```python
from build123d import *

# Parameters (mm, degrees)
SKETCH1_W           = 54
SKETCH1_H           = 44.4
SKETCH1_W_2         = 28
SKETCH1_H_2         = 6
BOSS_EXTRUDE1_DEPTH = 1.5
SKETCH2_R           = 1.5
SKETCH2_R_2         = 1
CUT_EXTRUDE1_DEPTH  = 1.5
BOSS_EXTRUDE2_DEPTH = 8
SKETCH4_R           = 7.5
BOSS_EXTRUDE3_DEPTH = 6
SKETCH5_R           = 5.877121991
BOSS_EXTRUDE4_DEPTH = 2
SKETCH6_R           = 7.5
BOSS_EXTRUDE5_DEPTH = 4
SKETCH7_R           = 5.097427656
CUT_EXTRUDE3_DEPTH  = 2
CHAMFER1_SIZE       = 2
BOSS_EXTRUDE6_DEPTH = 10
SKETCH9_W           = 9
SKETCH9_H           = 21
BOSS_EXTRUDE7_DEPTH = 10


with BuildPart() as part:
    # Sketch1 → Boss-Extrude1 (new body)
    with BuildSketch(Plane(origin=(0, 0, 0), x_dir=(1, 0, 0), z_dir=(0, 1, 0))):
        Rectangle(SKETCH1_W, SKETCH1_H)
        with Locations((0, -25.2)):
            Rectangle(SKETCH1_W_2, SKETCH1_H_2)
    extrude(amount=BOSS_EXTRUDE1_DEPTH)

    # Sketch2 → Cut-Extrude1 (cut)
    with BuildSketch(Plane(origin=(0, 1.5, 0), x_dir=(1, 0, 0), z_dir=(0, 1, 0))):
        with Locations(Location((-24, 19.2, 0), (0, 0, 270))):
            Circle(SKETCH2_R)
        with Locations(Location((24, 19.2, 0), (0, 0, 270))):
            Circle(SKETCH2_R)
        with Locations(Location((-24, -14.2, 0), (0, 0, 270))):
            Circle(SKETCH2_R)
        with Locations(Location((-10, -25.2, 0), (0, 0, 270))):
            Circle(SKETCH2_R)
        with Locations(Location((10, -25.2, 0), (0, 0, 270))):
            Circle(SKETCH2_R)
        with Locations(Location((0, 11.7, 0), (0, 0, 270))):
            Circle(SKETCH2_R_2)
    extrude(amount=-CUT_EXTRUDE1_DEPTH, mode=Mode.SUBTRACT)

    # Sketch3 → Boss-Extrude2 (add)
    with BuildSketch(Plane(origin=(0, 1.5, 0), x_dir=(1, 0, 0), z_dir=(0, 1, 0))):
        with BuildLine():
            Line((-8.5, 20.2), (8.5, 20.2))
            Line((8.5, 20.2), (8.5, 14.2))
            Line((8.5, 14.2), (11, 14.2))
            ThreePointArc((11, 14.2), (13.5, 11.7), (11, 9.2))
            Line((11, 9.2), (8.5, 9.2))
            Line((8.5, 9.2), (8.5, 3.2))
            Line((8.5, 3.2), (-8.5, 3.2))
            Line((-8.5, 3.2), (-8.5, 9.2))
            Line((-8.5, 9.2), (-11, 9.2))
            ThreePointArc((-11, 9.2), (-13.5, 11.7), (-11, 14.2))
            Line((-11, 14.2), (-8.5, 14.2))
            Line((-8.5, 14.2), (-8.5, 20.2))
        make_face()
    extrude(amount=BOSS_EXTRUDE2_DEPTH)

    # Sketch4 → Boss-Extrude3 (add)
    with BuildSketch(Plane(origin=(0, 9.5, 0), x_dir=(1, 0, 0), z_dir=(0, 1, 0))):
        with Locations(Location((0, 11.7, 0), (0, 0, 270))):
            Circle(SKETCH4_R)
    extrude(amount=BOSS_EXTRUDE3_DEPTH)

    # Sketch5 → Boss-Extrude4 (add)
    with BuildSketch(Plane(origin=(0, 15.5, 0), x_dir=(1, 0, 0), z_dir=(0, 1, 0))):
        with Locations(Location((0, 11.7, 0), (0, 0, 270))):
            Circle(SKETCH5_R)
    extrude(amount=BOSS_EXTRUDE4_DEPTH)

    # Sketch6 → Boss-Extrude5 (add)
    with BuildSketch(Plane(origin=(0, 17.5, 0), x_dir=(1, 0, 0), z_dir=(0, 1, 0))):
        with Locations(Location((0, 11.7, 0), (0, 0, 270))):
            Circle(SKETCH6_R)
    extrude(amount=BOSS_EXTRUDE5_DEPTH)

    # Sketch7 → Cut-Extrude3 (cut)
    with BuildSketch(Plane(origin=(0, 21.5, 0), x_dir=(1, 0, 0), z_dir=(0, 1, 0))):
        with Locations(Location((0, 11.7, 0), (0, 0, 270))):
            Circle(SKETCH7_R)
    extrude(amount=-CUT_EXTRUDE3_DEPTH, mode=Mode.SUBTRACT)

    # Chamfer1
    chamfer1_edges = [part.edges().sort_by_distance(p)[0] for p in [
        (0, 21.5, -16.797427656),
    ]]
    chamfer(chamfer1_edges, length=CHAMFER1_SIZE - 0.0001)  # a hair under: the kernel refuses the full size

    # Sketch8 → Boss-Extrude6 (add)
    with BuildSketch(Plane.XZ):
        Polygon((18, -7.2), (18, -15.2), (22, -14.2), (22, -8.2), align=None)
    extrude(amount=BOSS_EXTRUDE6_DEPTH)

    # Sketch9 → Boss-Extrude7 (add)
    with BuildSketch(Plane.XZ):
        with Locations((-18, -8.7)):
            Rectangle(SKETCH9_W, SKETCH9_H)
    extrude(amount=BOSS_EXTRUDE7_DEPTH)


solid = part.part
```
Input: part model. Units: mm. Frame: model coordinates. A direction names the side the tool comes from. Coordinates: 2 decimals unless noted, no trailing zeros. Write each loop counter-clockwise with the first axis right and the second up, starting at its lowest first coordinate (ties: lowest second). Pieces come first, ordered by that corner, then holes. Notation, with made-up numbers: (-25, 65) - (12, 65) arc R15 ccw to (12, 81) - close; hole circle Ø5 at (-33, 41.25). An arc over 180 degrees is marked (long way). Put each result on its own line as item: value. Start each with the question number.
1) Cut plane C-C (x = 10). Return the cut outline in (y, z), plus the area to 3 significant figures.
2) Reachability of faces 5 (the face through (20, -4.9, -7.7)), 6 (the face through (-8.5, 5, -17)), 7 (the face through (10, 5, -14.2)), 8 (the face through (0, 1.5, -12)) from +Z, -Z, +X, -X, +Y, -Y: full face, straight path, thin tool, end or side. Return the list, or none.
3) Cut plane B-B (y = -7.5). Return the cut outline in (x, z).
4) Ray query, L1, parallel to X at y = 0.7, z = 25.2; L2, parallel to X at y = 1, z = -19; L3, parallel to Y at x = -10, z = -15. Return the intervals inside material, ascending.
5) Contact query for flat-ended pins moving along their axis: pin 1 (0.8 mm diameter, centred on x = -9.5, y = 7, fed in from -Z); pin 2 (4.5 mm diameter, centred on x = -16, y = -7, fed in from -Z); pin 3 (3 mm diameter, centred on y = 4.5, z = -17.5, fed in from +X); pin 4 (8 mm diameter, centred on y = 10.5, z = 4.5, fed in from +X). Output: stop coordinate, or through.
6) Cut plane D-D (y = 7.5). Return the cut outline in (x, z).
7) Mould query, pull axis Z, two halves, no side actions, for faces 1 (the face through (-22.513, 0.76, -19.395)), 2 (the face through (0, 19.5, -12)), 3 (the face through (0, 5, -20.2)), 4 (the face through (-5, 15.5, -8)). Classes: pulls with the +Z half, pulls with the -Z half, needs draft (parallel to the pull), parting line crosses it, or undercut.
8) Cut plane A-A (x = -24). Return the cut outline in (y, z), plus the area to 3 significant figures.
Resolved:
1. outline: (0, -22.2) - (1.5, -22.2) - (1.5, -14.2) - (9.5, -14.2) - (9.5, -9.2) - (1.5, -9.2) - (1.5, 23.7) - (0, 23.7) - close; (0, 26.7) - (1.5, 26.7) - (1.5, 28.2) - (0, 28.2) - close
1. area: 111 mm2
2. face 5: +Z, +X, -Y
2. face 6: -Z, -X, +Y
2. face 7: -Z, +X, +Y
2. face 8: -Y
3. outline: (-22.5, -19.2) - (-13.5, -19.2) - (-13.5, 1.8) - (-22.5, 1.8) - close; (18, -15.2) - (22, -14.2) - (22, -8.2) - (18, -7.2) - close
4. L1: x = -14 to -11.5, -8.5 to 8.5, 11.5 to 14
4. L2: x = -27 to -25.49, -22.51 to 22.51, 25.49 to 27
4. L3: y = 0 to 1.5
5. pin 1: stops at z = -14.2
5. pin 2: stops at z = -19.2
5. pin 3: stops at x = 8.5
5. pin 4: passes through
6. outline: (-11, -14.2) - (-8.5, -14.2) - (-8.5, -20.2) - (8.5, -20.2) - (8.5, -14.2) - (11, -14.2) arc R2.5 ccw to (11, -9.2) - (8.5, -9.2) - (8.5, -3.2) - (-8.5, -3.2) - (-8.5, -9.2) - (-11, -9.2) arc R2.5 ccw to start
7. face 1: undercut
7. face 2: undercut
7. face 3: pulls with the -Z half
7. face 4: needs draft
8. outline: (0, -22.2) - (1.5, -22.2) - (1.5, -20.7) - (0, -20.7) - close; (0, -17.7) - (1.5, -17.7) - (1.5, 12.7) - (0, 12.7) - close; (0, 15.7) - (1.5, 15.7) - (1.5, 22.2) - (0, 22.2) - close
8. area: 57.6 mm2
